```python
from build123d import *

# Parameters (mm, degrees)
SKETCH1_W           = 34
SKETCH1_H           = 24
SKETCH1_W_2         = 23.744
SKETCH1_H_2         = 13.204
BOSS_EXTRUDE1_DEPTH = 2
SKETCH3_W           = 26.7
SKETCH3_H           = 22
CUT_EXTRUDE1_DEPTH  = 1.5
BOSS_EXTRUDE2_DEPTH = 0.8


with BuildPart() as part:
    # Sketch1 → Boss-Extrude1 (new body)
    with BuildSketch(Plane.XY):
        with Locations((-17, 12)):
            Rectangle(SKETCH1_W, SKETCH1_H)
        with Locations((-17.002, 11.998)):
            Rectangle(SKETCH1_W_2, SKETCH1_H_2, mode=Mode.SUBTRACT)
    extrude(amount=BOSS_EXTRUDE1_DEPTH)

    # Sketch3 → Cut-Extrude1 (cut)
    with BuildSketch(Plane(origin=(0, 0, 0), x_dir=(-1, 0, 0), z_dir=(0, 0, -1))):
        with Locations((17.002, 8.748)):
            Rectangle(SKETCH3_W, SKETCH3_H)
    extrude(amount=-CUT_EXTRUDE1_DEPTH, mode=Mode.SUBTRACT)

    # Sketch4 → Boss-Extrude2 (add)
    with BuildSketch(Plane(origin=(0, 0, 0), x_dir=(-1, 0, 0), z_dir=(0, 0, -1))):
        Polygon((1, 0), (-1, 0), (-1, 25), (0.739142899, 25), (35, 25), (35, 23.055979858), (35, 0), (33, 0), (33, 23), (1, 23), align=None)
    extrude(amount=BOSS_EXTRUDE2_DEPTH)


solid = part.part
```
Geometry: final body of the model. Coordinates: model frame, mm. A direction names the side the tool comes from. Round coordinates to 2 decimals unless told otherwise and drop trailing zeros. Order: outer loops, then holes, each group sorted by start corner. A loop starts at its lowest first (then second) coordinate and runs counter-clockwise, first axis right, second up. Notation, with made-up numbers: (-14, 25) - (25, 25) arc R20 ccw to (25, 47) - close; hole circle Ø3 at (7.25, -39). An arc over 180 degrees is marked (long way). Use CSV: the item, a comma, the result in double quotes. Start each with the question number.
Q1. Material intervals for line 1 along X through (y, z) = (7.75, 0.7); line 2 along X through (y, z) = (20.25, -0.6); line 3 along Y through (x, z) = (-8, 1.85), sorted ascending. Write a range as from..to.
Q2. Section query C-C (z = 1.1). Return loops of the section in (x, y), and give its area (3 significant figures).
Q3. Mould query, pull axis X, two halves, no side actions, for faces 4 (the face through (-14, 3, 1.5)), 5 (the face through (-30.352, 10, 1)), 6 (the face through (0, 12, 1)), 7 (the face through (-17, 24, 1)). Classes: +X half, -X half, draft (parallel to the pull), parting line (faces both ways), or undercut.
Q4. Section query D-D (y = 5). Return loops of the section in (x, z), and give its area (4 significant figures).
Q5. Section query B-B (y = 12). Return loops of the section in (x, z).
Q6. First-contact query: pin 1 (1.2 mm diameter, centred on x = -22, z = 0.5, fed in from -Y); pin 2 (0.6 mm diameter, centred on x = -15.5, z = 1.5, fed in from +Y); pin 3 (5 mm diameter, centred on x = -6.5, y = 17, fed in from -Z). Flat tips, straight axial feed; report the tip coordinate or a pass-through.
Q7. Access query for faces 1 (the face through (-18.4, 0, 1.7)), 2 (the face through (-34, 12, 1)), 3 (the face through (-3.652, 10, 1)). Directions: +Z, -Z, +X, -X, +Y, -Y. A direction counts if a zero-diameter tool reaches every point of the face in a straight line with its end or side. Return the directions, or none.
Q8. Section query A-A (x = -6). Return loops of the section in (y, z).
Result set:
1,line 1,"x = -34..-30.35, -3.65..0"
1,line 2,"x = -35..-33, -1..1"
1,line 3,"y = 0..5.4, 18.6..24"
2,outline,"(-34, 0) - (-30.35, 0) - (-30.35, 19.75) - (-3.65, 19.75) - (-3.65, 0) - (0, 0) - (0, 24) - (-34, 24) - close"
2,area,"289 mm2"
3,face 4,"undercut"
3,face 5,"undercut"
3,face 6,"+X half"
3,face 7,"draft"
4,outline,"(-35, -0.8) - (-33, -0.8) - (-33, 0) - (-30.35, 0) - (-30.35, 1.5) - (-3.65, 1.5) - (-3.65, 0) - (-1, 0) - (-1, -0.8) - (1, -0.8) - (1, 0) - (0, 0) - (0, 2) - (-34, 2) - (-34, 0) - (-35, 0) - close"
4,area,"31.15 mm2"
5,outline,"(-35, -0.8) - (-33, -0.8) - (-33, 0) - (-30.35, 0) - (-30.35, 1.5) - (-28.87, 1.5) - (-28.87, 2) - (-34, 2) - (-34, 0) - (-35, 0) - close; (-5.13, 1.5) - (-3.65, 1.5) - (-3.65, 0) - (-1, 0) - (-1, -0.8) - (1, -0.8) - (1, 0) - (0, 0) - (0, 2) - (-5.13, 2) - close"
6,pin 1,"stops at y = 19.75"
6,pin 2,"stops at y = 24"
6,pin 3,"stops at z = 1.5"
7,face 1,"+Z, -Z, +X, -X, -Y"
7,face 2,"+Z, -X, +Y, -Y"
7,face 3,"-Z, -Y"
8,outline,"(0, 1.5) - (5.4, 1.5) - (5.4, 2) - (0, 2) - close; (18.6, 1.5) - (19.75, 1.5) - (19.75, 0) - (23, 0) - (23, -0.8) - (25, -0.8) - (25, 0) - (24, 0) - (24, 2) - (18.6, 2) - close"
